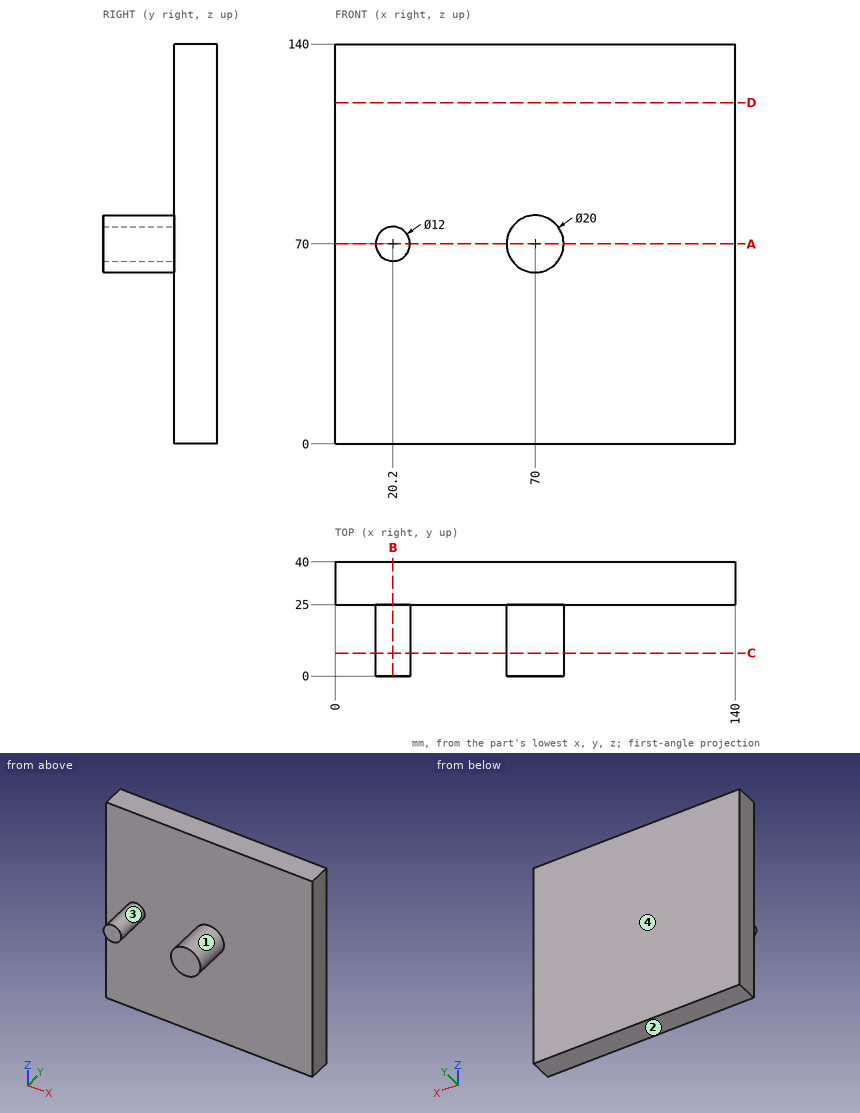
Answer from the drawing. Dimensions are ordinates in mm from the lowest x, y and z of the part. A direction names the side the tool comes from. Round coordinates to 2 decimals unless told otherwise and drop trailing zeros. Write each loop counter-clockwise with the first axis right and the second up, starting at its lowest first coordinate (ties: lowest second). Pieces come first, ordered by that corner, then holes. Notation, with made-up numbers: M 62.25,6.25 L 97.25,6.25 A28 ccw 97.25,27.25 Z; hole C -9.5,-8 d1. An arc over 180 degrees is marked long. One line per item, written item: value.
Q1. For a pull along X with two mould halves and no side action, classify the marked faces 3 and 4 as +X half, -X half, draft (parallel to the pull), parting line (faces both ways), or undercut.
Data:
face 3: undercut
face 4: draft
Q2. Find section D-D on z = 119.5. Write down the section's boundary in (x, y), plus the area to 3 significant figures.
Data:
outline: M 0,25 L 140,25 L 140,40 L 0,40 Z
area: 2,100 mm2
Q3. Flat-ended cylindrical pins translate along their axes: pin 1 Ø8 at (x, z) = (32.5, 31) entering from -Y; pin 2 Ø3 at (x, y) = (28.5, 8.5) entering from -Z; pin 3 Ø8 at (x, y) = (25.5, 7) entering from +Z. Find the tip coordinate at first contact, or state that the pin passes through.
Data:
pin 1: y = 25
pin 2: through
pin 3: z = 75.86
Q4. Find section B-B on x = 20.2. Write down the section's boundary in (y, z).
Data:
outline: M 0,64 L 25,64 L 25,0 L 40,0 L 40,140 L 25,140 L 25,76 L 0,76 Z
Q5. Find section C-C on y = 8. Write down the section's boundary in (x, z), plus the area to 3 significant figures.
Data:
outline: C 20.2,70 d12; C 70,70 d20
area: 427 mm2
Q6. Which of the six approach directions +Z, -Z, +X, -X, +Y, -Y give full straight-line access (tool end or side, diameter ignored) to the marked faces 1 and 2?
Data:
face 1: -Y
face 2: -Z, +X, -X, +Y, -Y
Q7. Straight lines are drawn through the part: line 1 (X direction, y = 3, z = 70.5); line 2 (Y direction, x = 16, z = 11.5); line 3 (Z direction, x = 25, y = 10.5). For each, find the intervals that lie inside material, in ascending order. Write a range as [from, to].
Data:
line 1: [14.22, 26.18], [60.01, 79.99]
line 2: [25, 40]
line 3: [66.4, 73.6]
Q8. Find section A-A on z = 70. Write down the section's boundary in (x, y).
Data:
outline: M 0,25 L 14.2,25 L 14.2,0 L 26.2,0 L 26.2,25 L 60,25 L 60,0 L 80,0 L 80,25 L 140,25 L 140,40 L 0,40 Z
